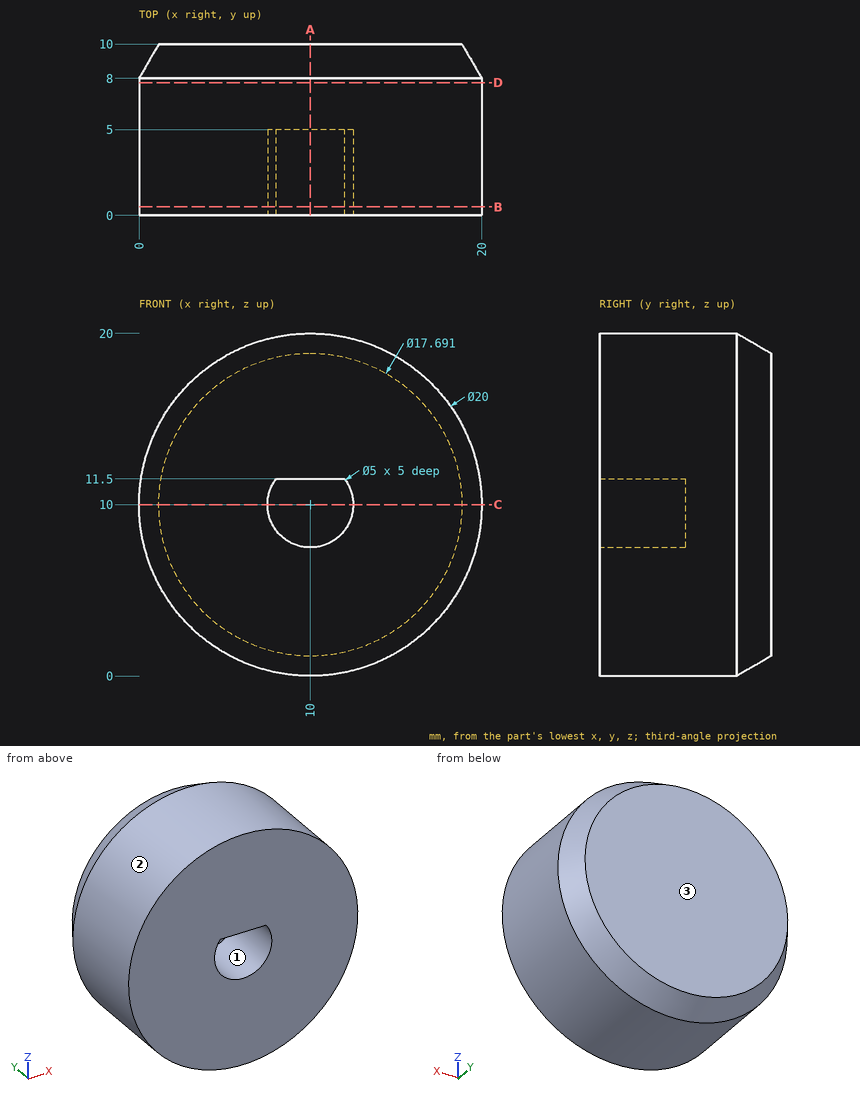
Check sheet for the drawn part. Datum: minimum x, y, z corner. Units: mm. Round coordinates to 2 decimals unless told otherwise and drop trailing zeros. Order: outer loops, then holes, each group sorted by start corner. A loop starts at its lowest first (then second) coordinate and runs counter-clockwise, first axis right, second up. Notation, with made-up numbers: M -39.5,38 L -35.5,38 A20 ccw -35.5,73 Z; hole C 72,-23.5 d4. An arc over 180 degrees is marked long. Answer in a Markdown table with one row per item.
(1) Material ranges on line 1 along X through (y, z) = (1.1, 10); line 2 along X through (y, z) = (7, 10.25); line 3 along Z through (x, y) = (8.5, 4) (1 decimal), recorded low to high. Write a range as from..to.
Findings:
| item | result |
|---|---|
| line 1 | x = 0..7.5, 12.5..20 |
| line 2 | x = 0..20 |
| line 3 | z = 0.1..8, 11.5..19.9 |
(2) Gauge pin test, flat ends, axial feed: pin 1 (1.5 mm diameter, centred on y = 2, z = 5, fed in from +X); pin 2 (4 mm diameter, centred on y = 9, z = 12.5, fed in from +X); pin 3 (3 mm diameter, centred on x = 11, z = 10.5, fed in from -Y); pin 4 (6 mm diameter, centred on x = 18, y = 4.5, fed in from -Z). Record the tip position at first contact, or that the pin passes through.
Findings:
| item | result |
|---|---|
| pin 1 | stops at x = 19.05 |
| pin 2 | stops at x = 19.97 |
| pin 3 | stops at y = 0 |
| pin 4 | stops at z = 1.34 |
(3) Section check C-C on z = 10. Record the boundary of the cut face in (x, y) (1 decimal), plus the area to 3 significant figures.
Findings:
| item | result |
|---|---|
| outline | M 0,0 L 7.5,0 L 7.5,5 L 12.5,5 L 12.5,0 L 20,0 L 20,8 L 18.8,10 L 1.2,10 L 0,8 Z |
| area | 173 mm^2 |
(4) Draft check along X on the marked faces 1, 2 and 3. Enter one of: +X half, -X half, draft (parallel to the pull), parting line (faces both ways), or undercut.
Findings:
| item | result |
|---|---|
| face 1 | undercut |
| face 2 | parting line |
| face 3 | draft |
(5) Section check B-B on y = 0.5. Record the boundary of the cut face in (x, z).
Findings:
| item | result |
|---|---|
| outline | C 10,10 d20; hole M 8,11.5 A2.5 ccw long 12,11.5 Z |
(6) Section check D-D on y = 7.75. Record the boundary of the cut face in (x, z), plus the area to 3 significant figures.
Findings:
| item | result |
|---|---|
| outline | C 10,10 d20 |
| area | 314 mm^2 |
(7) Section check A-A on x = 10. Record the boundary of the cut face in (y, z) (1 decimal).
Findings:
| item | result |
|---|---|
| outline | M 0,0 L 8,0 L 10,1.2 L 10,18.8 L 8,20 L 0,20 L 0,11.5 L 5,11.5 L 5,7.5 L 0,7.5 Z |
